Geometry: final body of the model. Coordinates: model frame, mm. A direction names the side the tool comes from. Give positions to 0.01 mm unless a question says otherwise; leave off trailing zeros. Order: outer loops, then holes, each group sorted by start corner. A loop starts at its lowest first (then second) coordinate and runs counter-clockwise, first axis right, second up. Notation, with made-up numbers: (83, -26.5) -> (89, -26.5) arc R17 cw to (89, -15.5) -> close; hole circle Ø2 at (-8, 65). An arc over 180 degrees is marked (long way). One line per question, with ' | ' between items. Start each with the question number.
(1) Section D-D (y = 1.75). Return loops of the section in (x, z) (3 decimals), then the cut area to 3 significant figures.
(2) Section C-C (x = -66). Return loops of the section in (y, z) (3 decimals).
(3) Section A-A (y = 19.05). Return loops of the section in (x, z), then the cut area to 3 significant figures.
(4) Ray query, L1, parallel to X at y = 19.05, z = -18.1; L2, parallel to X at y = 2.75, z = -1.25; L3, parallel to Z at x = 6.5, y = 23.25. Return the intervals inside material, ascending.
(5) Mould query, pull axis Y, two halves, no side actions, for faces 3 (the face through (-24.816, 16.117, -17.309)), 4 (the face through (-74.029, 16.117, -17.309)), 5 (the face through (-36, 14, -15.699)), 6 (the face through (-38, 25.4, -17)). Classes: +Y half, -Y half, draft (parallel to the pull), parting line (faces both ways), or undercut.
(6) Set-up query: faces 1 (the face through (-36, 0, -6)), 2 (the face through (-36, 3.175, -4)). Return all of +Z, -Z, +X, -X, +Y, -Y with unobstructed straight access to the full face (end or side cutting, diameter ignored); none if empty.
(7) Section B-B (z = 2). Return loops of the section in (x, y) (3 decimals), then the cut area to 3 significant figures.
(8) First-contact query: pin 1 Ø8.5 at (x, y) = (-51.43, 19.05) entering from +Z; pin 2 Ø8.5 at (x, z) = (0.96, 0.18) entering from +Y (3 decimals). Flat tips, straight axial feed; report the tip coordinate or a pass-through.
Autodesk Inventor part; units mm, degrees
ref_plane "YZ Plane" through (0, 0, 0) normal (1, 0, 0) x (0, 1, 0)
ref_plane "XZ Plane" through (0, 0, 0) normal (0, 1, 0) x (-1, 0, 0)
ref_plane "XY Plane" through (0, 0, 0) normal (0, 0, 1) x (1, 0, 0)
sketch "Sketch1" plane through (0, 0, 0) normal (0, 1, 0) x (-1, 0, 0)
  line L0 (-13.6552, 6.526) -> (87.9448, 6.526)
  line L1 (87.9448, 6.526) -> (87.9448, -18.874)
  line L2 (87.9448, -18.874) -> (-13.6552, -18.874)
  line L3 (-13.6552, -18.874) -> (-13.6552, 6.526)
  dimension "d0" = 101.6
  dimension "d1" = 25.4
extrude "Extrusion1" add sketch "Sketch1" along normal blind 3.175
sketch "Sketch2" plane through (0, 3.175, 0) normal (0, 1, 0) x (1, 0, 0)
  line L0 (-87.9448, 18.874) -> (13.6552, 18.874)
  line L1 (13.6552, 18.874) -> (13.6552, 15.699)
  line L2 (13.6552, 15.699) -> (-87.9448, 15.699)
  line L3 (-87.9448, 15.699) -> (-87.9448, 18.874)
  dimension "d4" = 101.6
  dimension "d5" = 3.175
extrude "Extrusion2" add sketch "Sketch2" along normal blind 22.225
sketch "Sketch3" plane through (0, 3.175, 0) normal (0, 1, 0) x (1, 0, 0)
  line L0 (-87.9448, 15.699) -> (-87.9448, -6.526)
  line L1 (-87.9448, -6.526) -> (13.6552, -6.526)
  line L2 (13.6552, -6.526) -> (13.6552, 15.699)
  point P0 (-75.2448, -0.176)
  point P1 (0.9552, -0.176)
  dimension "d8" = 12.7
  dimension "d9" = 12.7
  dimension "d10" = 6.35
hole "Hole1" at (-75.2448, 3.175, 0.176) at (0.9552, 3.175, 0.176) direction (0, -1, 0) diameter 6.35 end through all
sketch "Sketch4" plane through (-87.9448, 3.175, -15.699) normal (0, 0, 1) x (1, 0, 0)
  line L0 (0, 22.225) -> (101.6, 22.225)
  line L1 (101.6, 0) -> (101.6, 22.225)
  line L2 (0, 0) -> (0, 22.225)
  point P0 (12.7, 15.875)
  point P1 (88.9, 15.875)
  point P2 (61.9125, 15.875)
  point P3 (36.5125, 15.875)
  dimension "d18" = 6.35
  dimension "d26" = 39.6875
  dimension "d27" = 36.5125
hole "Hole2" at (-75.2448, 19.05, -15.699) at (0.9552, 19.05, -15.699) at (-51.4323, 19.05, -15.699) at (-26.0323, 19.05, -15.699) direction (0, 0, -1) diameter 6.35 end through all
properties part number "Connection to frame"
Response:
1) outline: (-87.945, -18.874) -> (13.655, -18.874) -> (13.655, 6.526) -> (-87.945, 6.526) -> close; hole circle Ø6.35 at (-75.245, 0.176); hole circle Ø6.35 at (0.955, 0.176) | area: 2,520 mm^2
2) outline: (0, -18.874) -> (25.4, -18.874) -> (25.4, -15.699) -> (3.175, -15.699) -> (3.175, 6.526) -> (0, 6.526) -> close
3) outline: (-87.94, -18.87) -> (-78.42, -18.87) -> (-78.42, -15.7) -> (-87.94, -15.7) -> close; (-72.07, -18.87) -> (-54.61, -18.87) -> (-54.61, -15.7) -> (-72.07, -15.7) -> close; (-48.26, -18.87) -> (-29.21, -18.87) -> (-29.21, -15.7) -> (-48.26, -15.7) -> close; (-22.86, -18.87) -> (-2.22, -18.87) -> (-2.22, -15.7) -> (-22.86, -15.7) -> close; (4.13, -18.87) -> (13.66, -18.87) -> (13.66, -15.7) -> (4.13, -15.7) -> close | area: 242 mm^2
4) L1: x = -87.94 to -78.42, -72.07 to -54.61, -48.26 to -29.21, -22.86 to -2.22, 4.13 to 13.66 | L2: x = -87.94 to -78.08, -72.41 to -1.88, 3.79 to 13.66 | L3: z = -18.87 to -15.7
5) face 3: undercut | face 4: undercut | face 5: draft | face 6: +Y half
6) face 1: +Z, -Z, +X, -X, -Y | face 2: +Z, +X, -X, +Y
7) outline: (-87.945, 0) -> (-77.844, 0) -> (-77.844, 3.175) -> (-87.945, 3.175) -> close; (-72.646, 0) -> (-1.644, 0) -> (-1.644, 3.175) -> (-72.646, 3.175) -> close; (3.554, 0) -> (13.655, 0) -> (13.655, 3.175) -> (3.554, 3.175) -> close | area: 290 mm^2
8) pin 1: stops at z = -15.7 | pin 2: stops at y = 3.175
